from build123d import *

# Parameters (mm, degrees)
SKETCH_R           = 10.5
SKETCH_W           = 6.6
SKETCH_H           = 6.6
PAD_DEPTH          = 10
POCKET001_DEPTH    = 72.674758
POLARPATTERN_COUNT = 9


with BuildPart() as part:
    # Sketch → Pad (new body)
    with BuildSketch(Plane.XY):
        Circle(SKETCH_R)
        Rectangle(SKETCH_W, SKETCH_H, mode=Mode.SUBTRACT)
    extrude(amount=PAD_DEPTH)

    # Sketch002 → Pocket001 (cut, through all)
    with BuildSketch(Plane.XY.offset(10)):
        with BuildLine():
            ThreePointArc((10.067451, -2.982687), (13.513887, -1e-06), (10.067452, 2.982686))
            ThreePointArc((9.547792, 1.707898), (10.03134, 2.254095), (10.067452, 2.982686))
            ThreePointArc((9.547792, 1.707898), (8.813944, 0.990369), (8.544593, 0))
            ThreePointArc((8.544593, 0), (8.813944, -0.990369), (9.547792, -1.707898))
            ThreePointArc((10.067451, -2.982687), (10.03134, -2.254096), (9.547792, -1.707898))
        make_face()
    pocket001 = extrude(amount=-POCKET001_DEPTH, mode=Mode.SUBTRACT)

    # PolarPattern: Pocket001 ×9 about axis
    polarpattern_axis = Axis((0, 0, 10), (0, 0, 1))
    for i in range(1, POLARPATTERN_COUNT):
        add(pocket001.rotate(polarpattern_axis, i * 360 / POLARPATTERN_COUNT), mode=Mode.SUBTRACT)


solid = part.part
Input: part model. Units: mm. Frame: model coordinates. A direction names the side the tool comes from. Round coordinates to 2 decimals unless told otherwise and drop trailing zeros. Order: outer loops, then holes, each group sorted by start corner. A loop starts at its lowest first (then second) coordinate and runs counter-clockwise, first axis right, second up. Notation, with made-up numbers: (74, -3) - (95, -3) arc R19 cw to (95, 6) - close; hole circle Ø3 at (34, 2.25). An arc over 180 degrees is marked (long way). Answer as a JSON object with one key per item and string values. Group by question number.
(1) Cut plane C-C (y = -6.5). Return loops of the section in (x, z).
(2) Pin query (flat end, axial travel): P1, Ø5.5, axis at y = 1.5, z = 7, coming from the +X side; P2, Ø2, axis at x = 7.5, z = 6.5, coming from the +Y side; P3, Ø1, axis at y = 5, z = 7, coming from the -X side. Return the tip coordinate at first contact, or that it passes through.
(3) Cut plane B-B (x = -9). Return loops of the section in (y, z), then the cut area to 3 significant figures.
(4) Reachability of faces 4 (the face through (4, 0, 10)), 5 (the face through (0, 3.3, 5)) from +Z, -Z, +X, -X, +Y, -Y: full face, straight path, thin tool, end or side. Return the list, or none.
(5) Material intervals for probe 1 along Y at (x, z) = (-8.5, 2); probe 2 along Y at (x, z) = (1.5, 1.5); probe 3 along X at (y, z) = (0.5, 5.5), sorted ascending. Write a range as from..to.
(6) Cut plane A-A (x = -3). Return loops of the section in (y, z).
(7) Draft query along Y for faces 1 (the face through (-0.469, 10.265, 5.07)), 2 (the face through (-3.3, 0, 5)), 3 (the face through (-10.5, 0, 4.9)). Return one class per face: released by +Y, released by -Y, zero draft, split by the parting line, or undercut.
Here are the results:
{
 "1": {"outline": "(-8.25, 0) - (6.1, 0) - (6.1, 10) - (-8.25, 10) - close"},
 "2": {"P1": "stops at x = 10.11", "P2": "stops at y = 5.55", "P3": "stops at x = -8.65"},
 "3": {"outline": "(-1.84, 0) - (1.84, 0) - (1.84, 10) - (-1.84, 10) - close", "area": "36.8 mm^2"},
 "4": {"face 4": "+Z, +X, -X, +Y, -Y", "face 5": "+Z, -Z"},
 "5": {"probe 1": "y = -6.16..-5.03, -2.19..2.19, 5.03..6.16", "probe 2": "y = -8.41..-3.3, 3.3..8.41", "probe 3": "x = -10.49..-3.3, 3.3..8.61"},
 "6": {"outline": "(-9.89, 0) - (-3.3, 0) - (-3.3, 10) - (-9.89, 10) - close; (3.3, 0) - (9.89, 0) - (9.89, 10) - (3.3, 10) - close"},
 "7": {"face 1": "released by +Y", "face 2": "undercut", "face 3": "split by the parting line"}
}
